Geometry: final body of the model. Coordinates: model frame, mm. Face numbers are marked on the shaded views. A direction names the side the tool comes from. Give positions to 0.01 mm unless a question says otherwise; leave off trailing zeros. Loops run counter-clockwise (first coordinate to the right, second up) from the corner with the lowest first, then second, coordinate; pieces in that order, holes last.
1. Draft query along Z for the marked faces 1, 2 and 3. Return one class per face: +Z half, -Z half, draft (parallel to the pull), parting line (faces both ways), or undercut.
2. Material intervals for line 1 along X through (y, z) = (-15.5, 44.45); line 2 along Y through (x, z) = (-50.55, 43); line 3 along Z through (x, y) = (-27.5, 6.5), sorted ascending.
3. Access query for the marked faces 4, 5, 6, 7 and 8. Directions: +Z, -Z, +X, -X, +Y, -Y. A direction counts if a zero-diameter tool reaches every point of the face in a straight line with its end or side. Return the directions, or none.
4. Section D-D, the plane z = 10.5. Output: boundary loops of the cut face in (x, y), then the cut area to 3 significant figures.
5. First-contact query: P1, Ø5.5, axis at y = -24.5, z = 41, coming from the -X side; P2, Ø5, axis at x = -31.5, z = 23.5, coming from the +Y side; P3, Ø0.9, axis at x = -20, y = 16, coming from the -Z side; P4, Ø8, axis at x = -44, z = -4, coming from the +Y side. Flat tips, straight axial feed; report the tip coordinate or a pass-through.
6. Section A-A, the plane z = 29.5. Output: boundary loops of the cut face in (x, y), then the cut area to 3 significant figures.
7. Section C-C, the plane x = -19.55. Output: boundary loops of the cut face in (y, z), then the cut area to 3 significant figures.
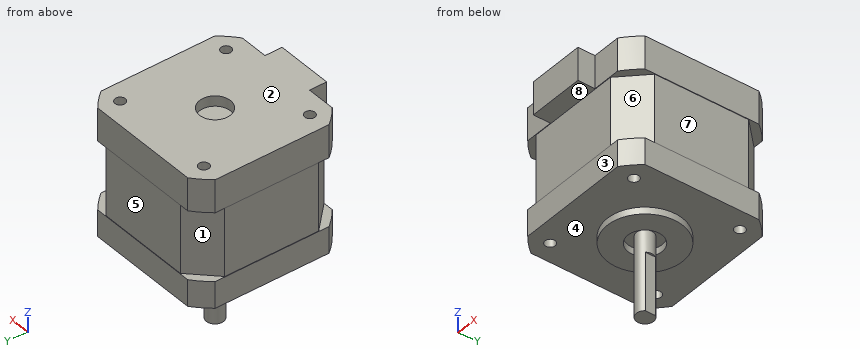
from build123d import *

# Parameters (mm, degrees)
PAD009_DEPTH              = 7.75
PAD010_DEPTH              = 20
PAD011_DEPTH              = 9.6
SKETCH017_R               = 1.5
POCKET004_DEPTH           = 4.5
SKETCH018_R               = 11
SKETCH018_R_2             = 5
PAD012_DEPTH              = 2
SKETCH019_R               = 2.5
PAD013_DEPTH              = 23.5
SKETCH020_W               = 0.5
SKETCH020_H               = 3
POCKET005_DEPTH           = 17
SKETCH021_R               = 1.5
SKETCH021_R_2             = 4.5
POCKET006_DEPTH           = 3
SKETCH022_W               = 16.5
SKETCH022_H               = 9.6
PAD014_DEPTH              = 5
CLONEBODY_PLACEMENT_ANGLE = 180


with BuildPart() as part:
    # Sketch014 → Pad009 (new body)
    with BuildSketch(Plane.XY):
        with BuildLine():
            Line((-16.65, -21.15), (16.65, -21.15))
            ThreePointArc((16.65, -21.15), (19.033457, -19.033457), (21.15, -16.65))
            Line((21.15, -16.65), (21.15, 16.65))
            ThreePointArc((21.15, 16.65), (19.033457, 19.033457), (16.65, 21.15))
            Line((16.65, 21.15), (-16.65, 21.15))
            ThreePointArc((-16.65, 21.15), (-19.033457, 19.033457), (-21.15, 16.65))
            Line((-21.15, 16.65), (-21.15, -16.65))
            ThreePointArc((-21.15, -16.65), (-19.033457, -19.033457), (-16.65, -21.15))
        make_face()
    extrude(amount=-PAD009_DEPTH)

    # Sketch015 (on Face10 of Pad009) → Pad010 (join)
    with BuildSketch(Plane(origin=(0, 0, -7.75), x_dir=(1, 0, 0), z_dir=(0, 0, -1))):
        Polygon((-21, -13.75), (-21, 13.75), (-13.75, 21), (13.75, 21), (21, 13.75), (21, -13.75), (13.75, -21), (-13.75, -21), align=None)
    extrude(amount=PAD010_DEPTH)

    # Sketch016 (on Face19 of Pad010) → Pad011 (join)
    with BuildSketch(Plane(origin=(0, 0, -27.75), x_dir=(1, 0, 0), z_dir=(0, 0, -1))):
        with BuildLine():
            Line((-16.65, -21.15), (16.65, -21.15))
            ThreePointArc((16.65, -21.15), (19.033457, -19.033457), (21.15, -16.65))
            Line((21.15, -16.65), (21.15, 16.65))
            ThreePointArc((21.15, 16.65), (19.033457, 19.033457), (16.65, 21.15))
            Line((16.65, 21.15), (-16.65, 21.15))
            ThreePointArc((-16.65, 21.15), (-19.033457, 19.033457), (-21.15, 16.65))
            Line((-21.15, 16.65), (-21.15, -16.65))
            ThreePointArc((-21.15, -16.65), (-19.033457, -19.033457), (-16.65, -21.15))
        make_face()
    extrude(amount=PAD011_DEPTH)

    # Sketch017 (on Face4 of Pad011) → Pocket004 (cut)
    with BuildSketch(Plane.XY):
        with Locations((-15.5, 15.5)):
            Circle(SKETCH017_R)
        with Locations((15.5, 15.5)):
            Circle(SKETCH017_R)
        with Locations((15.5, -15.5)):
            Circle(SKETCH017_R)
        with Locations((-15.5, -15.5)):
            Circle(SKETCH017_R)
    extrude(amount=-POCKET004_DEPTH, mode=Mode.SUBTRACT)

    # Sketch018 (on Face4 of Pocket004) → Pad012 (join)
    with BuildSketch(Plane.XY):
        Circle(SKETCH018_R)
        Circle(SKETCH018_R_2, mode=Mode.SUBTRACT)
    extrude(amount=PAD012_DEPTH)

    # Sketch019 (on Face39 of Pad012) → Pad013 (join)
    with BuildSketch(Plane.XY):
        Circle(SKETCH019_R)
    extrude(amount=PAD013_DEPTH)

    # Sketch020 (on Face42 of Pad013) → Pocket005 (cut)
    with BuildSketch(Plane.XY.offset(23.5)):
        with Locations((-2.25, 0)):
            Rectangle(SKETCH020_W, SKETCH020_H)
    extrude(amount=-POCKET005_DEPTH, mode=Mode.SUBTRACT)

    # Sketch021 (on Face40 of Pocket005) → Pocket006 (cut)
    with BuildSketch(Plane(origin=(0, 0, -37.35), x_dir=(1, 0, 0), z_dir=(0, 0, -1))):
        with Locations((-15.5, 15.5)):
            Circle(SKETCH021_R)
        with Locations((15.5, 15.5)):
            Circle(SKETCH021_R)
        with Locations((15.5, -15.5)):
            Circle(SKETCH021_R)
        with Locations((-15.5, -15.5)):
            Circle(SKETCH021_R)
        Circle(SKETCH021_R_2)
    extrude(amount=-POCKET006_DEPTH, mode=Mode.SUBTRACT)

    # Sketch022 (on Face38 of Pocket006) → Pad014 (join)
    with BuildSketch(Plane.XZ.offset(21.15)):
        with Locations((0, -32.55)):
            Rectangle(SKETCH022_W, SKETCH022_H)
    extrude(amount=PAD014_DEPTH)


with BuildPart() as part_1:
    # CloneBody placement: moved
    add(part.part.moved(Location((-35.05, 0, 8))).rotate(Axis((-35.05, 0, 8), (0, 1, 0)), CLONEBODY_PLACEMENT_ANGLE))


solid = part_1.part
Answers below:
1. face 1: undercut
1. face 2: +Z half
1. face 3: draft
2. line 1: x = -56.2 to -52.05, -49.05 to -21.05, -18.05 to -13.9
2. line 2: y = -21.15 to -17, -14 to 14, 17 to 21.15
2. line 3: z = 6 to 45.35
3. face 4: -Z
3. face 5: +X, -X, +Y
3. face 6: +X, -Y
3. face 7: +X, +Y, -Y
3. face 8: none
4. outline: (-56.2, -16.65) arc R26.92 ccw to (-51.7, -21.15) - (-18.4, -21.15) arc R26.92 ccw to (-13.9, -16.65) - (-13.9, 16.65) arc R26.92 ccw to (-18.4, 21.15) - (-51.7, 21.15) arc R26.92 ccw to (-56.2, 16.65) - close; hole circle Ø3 at (-50.55, -15.5); hole circle Ø3 at (-50.55, 15.5); hole circle Ø3 at (-19.55, -15.5); hole circle Ø3 at (-19.55, 15.5)
4. area: 1,720 mm2
5. P1: stops at x = -43.3
5. P2: stops at y = 21
5. P3: stops at z = 12.5
5. P4: passes through
6. outline: (-56.05, -13.75) - (-48.8, -21) - (-21.3, -21) - (-14.05, -13.75) - (-14.05, 13.75) - (-21.3, 21) - (-48.8, 21) - (-56.05, 13.75) - close
6. area: 1,660 mm2
7. outline: (-21.15, 8) - (-17, 8) - (-17, 12.5) - (-14, 12.5) - (-14, 8) - (14, 8) - (14, 12.5) - (17, 12.5) - (17, 8) - (21.15, 8) - (21.15, 15.75) - (19.25, 15.75) - (19.25, 35.75) - (21.15, 35.75) - (21.15, 45.35) - (17, 45.35) - (17, 42.35) - (14, 42.35) - (14, 45.35) - (-14, 45.35) - (-14, 42.35) - (-17, 42.35) - (-17, 45.35) - (-21.15, 45.35) - (-21.15, 35.75) - (-19.25, 35.75) - (-19.25, 15.75) - (-21.15, 15.75) - close
7. area: 1,460 mm2
